For this review, take the finished solid that the model builds, in its own axes (mm). A direction names the side the tool comes from. Coordinates: 2 decimals unless noted, no trailing zeros. Order: outer loops, then holes, each group sorted by start corner. A loop starts at its lowest first (then second) coordinate and runs counter-clockwise, first axis right, second up. Notation, with made-up numbers: (-30.75, -28) -> (2.25, -28) arc R22 cw to (2.25, 3) -> close; hole circle Ø1 at (-20, 40.5). An arc over 180 degrees is marked (long way). Answer as a JSON object with one key per item and string values. Group by question number.
1) Add section C-C, the plane y = 15.75. Write out the cut boundary in (x, z).
2) Wall thickness on L1, parallel to X at y = 16.75, z = 0; L2, parallel to Z at x = 0, y = 12.25: over which ranges is each line inside the solid? List them lowest first.
3) For pin 1 (4 mm diameter, centred on y = 7.5, z = -3.5, fed in from +X); pin 2 (3 mm diameter, centred on x = -0.5, z = -2, fed in from -Y); pin 3 (3 mm diameter, centred on y = 5.5, z = -2.5, fed in from +X), all flat-tipped, find the tip position at first contact; note any pin that passes through.
4) Add section B-B, the plane x = 0. Write out the cut boundary in (y, z), then the cut area to 3 significant figures.
5) Add section D-D, the plane x = 3.75. Write out the cut boundary in (y, z), then the cut area to 3 significant figures.
6) Machinability: for faces 4 (the cylindrical face through (2.192, 7.395, -4.214)), 5 (the flat face through (3, 19, 3)), which of the approach directions +Z, -Z, +X, -X, +Y, -Y give a long, thin tool a straight path to every point of the face, cutting with its end or side? Answer none if there is none.
7) Add section A-A, the plane z = 0. Write out the cut boundary in (x, y), then the cut area to 3 significant figures.
8) Draft analysis for pull direction X (two halves, no side actions). For faces 1 (the flat face through (1, 0, -5)), 2 (the cylindrical face through (-1.46, 9.63, 6.59)), 3 (the flat face through (-4, 15, 0)), state which applies: +X half, -X half, draft (parallel to the pull), parting line (faces both ways), or undercut.
Autodesk Inventor part; units mm, degrees
ref_plane "YZ Plane" through (0, 0, 0) normal (1, 0, 0) x (0, 1, 0)
ref_plane "XZ Plane" through (0, 0, 0) normal (0, 1, 0) x (-1, 0, 0)
ref_plane "XY Plane" through (0, 0, 0) normal (0, 0, 1) x (1, 0, 0)
sketch "Sketch1" plane through (0, 0, 0) normal (0, 0, 1) x (1, 0, 0)
  line L0 (0, 0) -> (4.75, 0) construction
  line L1 (6.75, 0) -> (6.75, 19)
  line L2 (6.75, 19) -> (3.5, 19)
  line L3 (3.5, 19) -> (3.5, 15)
  line L4 (3.5, 15) -> (3.5, 15)
  line L5 (3.5, 15) -> (3.5, 5) construction
  line L6 (3.5, 5) -> (0, 5) construction
  line L7 (0, 5) -> (0, 0) construction
  line L8 (4.75, 5) -> (3.5, 5)
  line L9 (3.5, 5) -> (3.5, 10.822) construction
  line L10 (3.5, 15) -> (4.75, 15)
  line L11 (4.75, 15) -> (4.75, 5)
  line L12 (4.75, 5) -> (3.5, 5)
  line L13 (4.75, 5) -> (4.75, 0)
  line L14 (4.75, 0) -> (6.75, 0)
  line L15 (0, -3.8) -> (0, 22.8)
  point P0 (3.375, 0)
  dimension "d0" = 4
  dimension "d7" = 3.5
  dimension "d9" = 10
  dimension "d11" = 4.75
  dimension "d12" = 2
  dimension "d13" = 5
revolve "Revolution1" add sketch "Sketch1" angle 360 about axis through (0, -10, 0) along (0, 1, 0)
properties part number "ButtonHolder_V3_3DPrint"
Output values:
{
 "1": {"outline": "circle Ø13.5 at (0, 0); hole circle Ø7 at (0, 0)"},
 "2": {"L1": "x = -6.75 to -3.5, 3.5 to 6.75", "L2": "z = -6.75 to -4.75, 4.75 to 6.75"},
 "3": {"pin 1": "stops at x = 6.58", "pin 2": "stops at y = 15", "pin 3": "stops at x = 6.68"},
 "4": {"outline": "(0, -6.75) -> (19, -6.75) -> (19, -3.5) -> (15, -3.5) -> (15, -4.75) -> (0, -4.75) -> close; (0, 4.75) -> (15, 4.75) -> (15, 3.5) -> (19, 3.5) -> (19, 6.75) -> (0, 6.75) -> close", "area": "86.0 mm²"},
 "5": {"outline": "(0, -5.61) -> (19, -5.61) -> (19, 5.61) -> (0, 5.61) -> (0, 2.92) -> (15, 2.92) -> (15, -2.92) -> (0, -2.92) -> close", "area": "126 mm²"},
 "6": {"face 4": "-Y", "face 5": "+Z, -Z, +X, -X, +Y"},
 "7": {"outline": "(-6.75, 0) -> (-4.75, 0) -> (-4.75, 15) -> (-3.5, 15) -> (-3.5, 19) -> (-6.75, 19) -> close; (3.5, 15) -> (4.75, 15) -> (4.75, 0) -> (6.75, 0) -> (6.75, 19) -> (3.5, 19) -> close", "area": "86.0 mm²"},
 "8": {"face 1": "draft", "face 2": "parting line", "face 3": "undercut"}
}
